Work out the finished part from the listing and answer in its coordinate system (mm). A direction names the side the tool comes from. Round coordinates to 2 decimals unless told otherwise and drop trailing zeros. Loops run counter-clockwise (first coordinate to the right, second up) from the corner with the lowest first, then second, coordinate; pieces in that order, holes last.
Autodesk Inventor part; units mm, degrees
ref_plane "YZ Plane" through (0, 0, 0) normal (1, 0, 0) x (0, 1, 0)
ref_plane "XZ Plane" through (0, 0, 0) normal (0, 1, 0) x (-1, 0, 0)
ref_plane "XY Plane" through (0, 0, 0) normal (0, 0, 1) x (1, 0, 0)
sketch "スケッチ1" plane through (0, 0, 0) normal (0, 0, 1) x (1, 0, 0)
  line L0 (-22, -24) -> (22, -24)
  line L1 (22, -24) -> (22, 24)
  line L2 (22, 24) -> (-22, 24)
  line L3 (-22, 24) -> (-22, -24)
  line L4 (-22, -24) -> (22, 24) construction
  line L5 (22, -24) -> (-22, 24) construction
  line L6 (-17, 15) -> (17, 15)
  line L7 (17, 15) -> (17, -19)
  line L8 (17, -19) -> (-17, -19)
  line L9 (-17, -19) -> (-17, 15)
  circle A0 centre (-17, 15) radius 3
  circle A1 centre (17, 15) radius 3
  circle A2 centre (17, -19) radius 3
  circle A3 centre (-17, -19) radius 3
  circle A4 centre (-17, 15) radius 8
  circle A5 centre (17, 15) radius 8
  circle A6 centre (17, -19) radius 8
  circle A7 centre (-17, -19) radius 8
  line L10 (-22, -24) -> (22, -24)
  line L11 (22, -24) -> (22, -28)
  line L12 (22, -28) -> (-22, -28)
  line L13 (-22, -28) -> (-22, -24)
  line L14 (-2.5, 15) -> (2.5, 15)
  line L15 (2.5, 15) -> (2.5, -19)
  line L16 (2.5, -19) -> (-2.5, -19)
  line L17 (-2.5, -19) -> (-2.5, 15)
  line L18 (10.5, 15) -> (10.5, -19)
  line L19 (5.5, -19) -> (5.5, 15)
  line L20 (18.5, 15) -> (18.5, -19)
  line L21 (13.5, -19) -> (13.5, 15)
  line L22 (-5.5, 15) -> (-5.5, -19)
  line L23 (-10.5, -19) -> (-10.5, 15)
  line L24 (2.5, 15) -> (2.5, -19)
  line L25 (-2.5, -19) -> (-2.5, 15)
  line L26 (10.5, 15) -> (10.5, -19)
  line L27 (5.5, -19) -> (5.5, 15)
  line L28 (-13.5, 15) -> (-13.5, -19)
  line L29 (-18.5, -19) -> (-18.5, 15)
  line L30 (-5.5, 15) -> (-5.5, -19)
  line L31 (-10.5, -19) -> (-10.5, 15)
  line L32 (2.5, 15) -> (2.5, -19)
  line L33 (-2.5, -19) -> (-2.5, 15)
  point P0 (0, 0)
  point P1 (-9, 15)
  point P2 (9, 15)
  point P3 (17, 7)
  point P4 (17, -11)
  point P5 (9, -19)
  point P6 (-9, -19)
  point P7 (-17, -11)
  point P8 (-17, 7)
  point P9 (22, -24)
  point P10 (0, 15)
  point P11 (-18.5, 7.1419)
  point P12 (-18.5, -11.1419)
  point P13 (-13.5, -11.8063)
  point P14 (-13.5, 7.8063)
  point P15 (-10.5, 15)
  point P16 (-10.5, -19)
  point P17 (-5.5, -19)
  point P18 (-5.5, 15)
  point P19 (13.5, 7.8063)
  point P20 (13.5, -11.8063)
  point P21 (18.5, -11.1419)
  point P22 (18.5, 7.1419)
  point P23 (5.5, 15)
  point P24 (5.5, -19)
  point P25 (10.5, -19)
  point P26 (10.5, 15)
  point P27 (-2.5, -19)
  point P28 (2.5, 15)
  point P29 (-10.5, -14.3363)
  point P30 (-10.5, 10.3363)
  point P31 (10.5, 10.3363)
  point P32 (10.5, -14.3363)
  dimension "d0" = 48
  dimension "d1" = 44
  dimension "d2" = 34
  dimension "d3" = 5
  dimension "d4" = 5
  dimension "d5" = 6
  dimension "d6" = 16
  dimension "d11" = 4
  dimension "d12" = 5
  dimension "d15" = 8
  dimension "d18" = 8
extrude "プレート1" add sketch "スケッチ1" along normal blind 1.5 contours L3 A7 L29 A3 L8 L0 | L0 A7 L13 | A7 L8 A6 L0 | L0 A6 L11 L12 L13 A7 | L3 A4 L29 A7 | A6 L8 A2 L20 L1 L0 | L0 L11 A6 | L8 L23 A7 | L3 A4 L6 A0 L29 | A7 L9 A3 L29 | A6 L18 L8 | L22 L6 L17 L8 | L8 L28 A7 L23 | A7 L28 A4 L23 | L3 L2 L1 A5 L6 A4 | L29 A0 L9 A4 | A7 L28 L8 A3 L9 | A6 L20 A5 L1 | L18 A6 L21 L8 | L8 L15 L6 L19 | L18 A5 L21 A6 | L23 L6 A4 | A4 L28 L6 L23 | L9 A0 L6 L28 A4 | A5 L20 A1 L6 L1 | L20 A2 L7 A6 | L21 A6 L7 A2 L8 | L18 L6 L21 A5 | A5 L6 L18 | A5 L7 A1 L20 | L21 L6 A1 L7 A5
sketch "スケッチ2" plane through (0, 0, 1.5) normal (0, 0, 1) x (1, 0, 0)
  line L0 (11.5, -21.5) -> (11.5, -14.8)
  line L1 (11.5, -21.5) -> (12, -21.5)
  line L2 (12, -21.5) -> (12, -24)
  line L3 (18, -24) -> (14, -24)
  line L4 (18, -14) -> (18, -24) construction
  line L5 (12.3, -14) -> (18, -14)
  circle A0 centre (12.3, -14.8) radius 0.8
  circle A1 centre (14, -23.2) radius 0.8
  line L6 (0, 0) -> (0, -10)
  circle A2 centre (-12.3, -14.8) radius 0.8
  circle A3 centre (-14, -23.2) radius 0.8
  arc A4 (11.5, -14.8) -> (12.3, -14) centre (12.3, -14.8) ccw
  line L7 (14, -24) -> (12, -24)
  circle A5 centre (14, -23.2) radius 0.8
  dimension "d21" = 1.6
  dimension "d22" = 1.6
  dimension "d25" = 2
extrude "切り取り1" cut sketch "スケッチ2" against normal blind 1.5
sketch "スケッチ3" plane through (0, 0, 1.5) normal (0, 0, 1) x (1, 0, 0)
  circle A0 centre (0, 19) radius 0.8
  circle A1 centre (-10, 19) radius 0.8
  circle A2 centre (10, 19) radius 0.8
  line L0 (-22, 24) -> (22, 24)
  point P0 (0, 0)
  point P1 (0, 24)
  dimension "d26" = 1.6
  dimension "d27" = 1.6
  dimension "d28" = 1.6
  dimension "d29" = 5
  dimension "d30" = 10
  dimension "d31" = 10
extrude "切り取り2" cut sketch "スケッチ3" against normal blind 1.5
equation "\"d4\" = d3"
equation "\"d23\" = Thickness"
equation "\"d32\" = Thickness"
equation "\"d10\" = Thickness"
equation "\"BendRadius\" = Thickness"
equation "\"BendReliefWidth\" = Thickness"
equation "\"BendReliefDepth\" = 0.5 * Thickness"
equation "\"CornerReliefSize\" = 4 * Thickness"
equation "\"MinimumRemnant\" = 2 * Thickness"
equation "\"TransitionRadius\" = BendRadius"
equation "\"JacobiRadiusSize\" = BendRadius"
equation "\"GapSize\" = Thickness"
properties part number "board_setter_base" material "アルミニウム 6061"
1. Which of the six approach directions +Z, -Z, +X, -X, +Y, -Y give full straight-line access (tool end or side, diameter ignored) to faces 1 (the face through (9.374, -16.584, 0.74)), 2 (the face through (-5, -2, 1.5))?
Answer key:
face 1: +Z, -Z
face 2: +Z, +X, -X, +Y, -Y
2. Given pin 1 (8 mm diameter, centred on x = -17.5, y = 16, fed in from +Z), flat-ended and moving along its own axis, determine where the tip first touches the part or whether it passes through.
Answer key:
pin 1: stops at z = 1.5
3. Find section A-A (x = 0). Write down the section's boundary in (y, z).
Answer key:
outline: (-28, 0) - (-19, 0) - (-19, 1.5) - (-28, 1.5) - close; (15, 0) - (18.2, 0) - (18.2, 1.5) - (15, 1.5) - close; (19.8, 0) - (24, 0) - (24, 1.5) - (19.8, 1.5) - close
4. Find section B-B (y = 4). Write down the section's boundary in (x, z), then the cut area to 3 significant figures.
Answer key:
outline: (-22, 0) - (-18.5, 0) - (-18.5, 1.5) - (-22, 1.5) - close; (-13.5, 0) - (-10.5, 0) - (-10.5, 1.5) - (-13.5, 1.5) - close; (-5.5, 0) - (-2.5, 0) - (-2.5, 1.5) - (-5.5, 1.5) - close; (2.5, 0) - (5.5, 0) - (5.5, 1.5) - (2.5, 1.5) - close; (10.5, 0) - (13.5, 0) - (13.5, 1.5) - (10.5, 1.5) - close; (18.5, 0) - (22, 0) - (22, 1.5) - (18.5, 1.5) - close
area: 28.5 mm2
5. Determine the mould class of faces 3 (the face through (7, -19, 1)), 4 (the face through (0, 24, 1)), 5 (the face through (-22, -2, 1)) for opening direction X: +X half, -X half, draft (parallel to the pull), parting line (faces both ways), or undercut.
Answer key:
face 3: undercut
face 4: draft
face 5: -X half
6. Consider probe 1 along X at (y, z) = (1, 0.65); probe 2 along Y at (x, z) = (17, 1.05); probe 3 along Y at (x, z) = (0, 1.1). Determine where each line is inside the solid, lowest interval first.
Answer key:
probe 1: x = -22 to -18.5, -13.5 to -10.5, -5.5 to -2.5, 2.5 to 5.5, 10.5 to 13.5, 18.5 to 22
probe 2: y = -28 to -22, -16 to -11, 7 to 12, 18 to 24
probe 3: y = -28 to -19, 15 to 18.2, 19.8 to 24
7. Find section D-D (x = -12.3). Write down the section's boundary in (y, z), then the cut area to 3 significant figures.
Answer key:
outline: (-28, 0) - (-15.6, 0) - (-15.6, 1.5) - (-28, 1.5) - close; (-14, 0) - (24, 0) - (24, 1.5) - (-14, 1.5) - close
area: 75.6 mm2
8. Find section C-C (y = -23.2). Write down the section's boundary in (x, z).
Answer key:
outline: (-22, 0) - (-14.8, 0) - (-14.8, 1.5) - (-22, 1.5) - close; (-13.2, 0) - (13.2, 0) - (13.2, 1.5) - (-13.2, 1.5) - close; (14.8, 0) - (22, 0) - (22, 1.5) - (14.8, 1.5) - close
